Autodesk Inventor part; units mm, degrees
ref_plane "YZ Plane" through (0, 0, 0) normal (1, 0, 0) x (0, 1, 0)
ref_plane "XZ Plane" through (0, 0, 0) normal (0, 1, 0) x (-1, 0, 0)
ref_plane "XY Plane" through (0, 0, 0) normal (0, 0, 1) x (1, 0, 0)
sketch "BaseBottom" plane through (0, 0, 0) normal (0, 1, 0) x (-1, 0, 0)
  line L0 (108.8151, 0.0203) -> (-41.1849, 0.0203)
  line L1 (-46.1849, -4.9797) -> (-46.1849, -74.9797)
  line L2 (-41.1849, -79.9797) -> (108.8151, -79.9797)
  line L3 (113.8151, -74.9797) -> (113.8151, -4.9797)
  arc A0 (113.8151, -4.9797) -> (108.8151, 0.0203) centre (108.8151, -4.9797) ccw
  arc A1 (108.8151, -79.9797) -> (113.8151, -74.9797) centre (108.8151, -74.9797) ccw
  arc A2 (-46.1849, -74.9797) -> (-41.1849, -79.9797) centre (-41.1849, -74.9797) ccw
  arc A3 (-41.1849, 0.0203) -> (-46.1849, -4.9797) centre (-41.1849, -4.9797) ccw
  line L4 (109.3151, -1.9797) -> (-41.6849, -1.9797)
  line L5 (-44.1849, -4.4797) -> (-44.1849, -75.4797)
  line L6 (-41.6849, -77.9797) -> (109.3151, -77.9797)
  line L7 (111.8151, -75.4797) -> (111.8151, -4.4797)
  arc A4 (-41.6849, -1.9797) -> (-44.1849, -4.4797) centre (-41.6849, -4.4797) ccw
  arc A5 (-44.1849, -75.4797) -> (-41.6849, -77.9797) centre (-41.6849, -75.4797) ccw
  arc A6 (109.3151, -77.9797) -> (111.8151, -75.4797) centre (109.3151, -75.4797) ccw
  arc A7 (111.8151, -4.4797) -> (109.3151, -1.9797) centre (109.3151, -4.4797) ccw
  line L8 (-46.1849, -29.9797) -> (-44.1849, -29.9797)
  line L9 (-44.1849, -29.9797) -> (-44.1849, -49.9797)
  line L10 (-44.1849, -49.9797) -> (-46.1849, -49.9797)
  line L11 (-46.1849, -49.9797) -> (-46.1849, -29.9797)
  point P0 (-46.1849, -79.9797)
  point P1 (-46.1849, 0.0203)
  point P2 (113.8151, -79.9797)
  point P3 (-44.1849, -77.9797)
  point P4 (-44.1849, -1.9797)
  point P5 (111.8151, -77.9797)
  point P6 (-45.1849, -49.9797)
  dimension "d2" = 160
  dimension "d3" = 80
  dimension "d4" = 5
  dimension "d6" = 156
  dimension "d7" = 76
  dimension "d8" = 2
  dimension "d9" = 2
  dimension "d10" = 2.5
  dimension "d11" = 20
  dimension "d12" = 30
extrude "BaseFloor" add sketch "BaseBottom" against normal blind 2
extrude "BaseFill" add sketch "BaseBottom" along normal blind 98
extrude "BaseHollow" cut sketch "BaseBottom" along normal blind 100 contours L5 A4 L4 A7 L7 A6 L6 A5
properties part number "Base"
Can you work these out from the model? Positions are in its coordinate system, mm. A direction names the side the tool comes from. Give positions to 0.01 mm unless a question says otherwise; leave off trailing zeros. Write each loop counter-clockwise with the first axis right and the second up, starting at its lowest first coordinate (ties: lowest second). Pieces come first, ordered by that corner, then holes. Notation, with made-up numbers: (44.5, 28.5) -> (97.5, 28.5) arc R21 ccw to (97.5, 47.5) -> close; hole circle Ø9 at (35, 14). An arc over 180 degrees is marked (long way). Answer as a JSON object with one key per item and string values. Group by question number.
Item 1: For faces 1 (the face through (-112.389, 48.7, -1.483)), 2 (the face through (44.185, 48, -39)), which set-ups out of +Z, -Z, +X, -X, +Y, -Y let a thin tool reach every point of the face, with its end or its side?
Item 2: Suppose I cut it at A-A (y = 74.5). Please give me the cut outline in (x, z), plus the area to 3 significant figures.
Item 3: Please list where these lines run through material, in increasing order: line 1 (X direction, y = 32.5, z = -53); line 2 (Z direction, x = -41.5, y = 57); line 3 (Y direction, x = -79, z = -74.5). Write a range as [from, to].
Item 4: Suppose I cut it at B-B (z = -56). Please give me the cut outline in (x, y), plus the area to 3 significant figures.
Item 5: We'd pull the mould along Z, two halves only. Please class faces 3 (the face through (-113.815, 49, -40)), 4 (the face through (-33, 48, -77.98)), 5 (the face through (-112.312, 48.7, -78.554)): +Z half, -Z half, draft (parallel to the pull), parting line (faces both ways), or undercut.
Item 6: Suppose I cut it at C-C (x = -100). Please give me the cut outline in (y, z).
Item 7: I'm going to push a flat-ended pin straight in: P1, Ø2, axis at x = -4.5, z = -13, coming from the +Y side. Where does the tip first touch, or does it pass through?
Findings:
{
 "1": {"face 1": "+Z, -X, +Y, -Y", "face 2": "+Y"},
 "2": {"outline": "(-113.82, -74.98) arc R5 ccw to (-108.82, -79.98) -> (41.18, -79.98) arc R5 ccw to (46.18, -74.98) -> (46.18, -4.98) arc R5 ccw to (41.18, 0.02) -> (-108.82, 0.02) arc R5 ccw to (-113.82, -4.98) -> close; hole (-111.82, -75.48) arc R2.5 ccw to (-109.32, -77.98) -> (41.68, -77.98) arc R2.5 ccw to (44.18, -75.48) -> (44.18, -4.48) arc R2.5 ccw to (41.68, -1.98) -> (-109.32, -1.98) arc R2.5 ccw to (-111.82, -4.48) -> close", "area": "928 mm²"},
 "3": {"line 1": "x = [-113.82, -111.82], [44.18, 46.18]", "line 2": "z = [-79.98, -77.98], [-1.98, 0.02]", "line 3": "y = [-2, 0]"},
 "4": {"outline": "(-113.82, -2) -> (46.18, -2) -> (46.18, 98) -> (44.18, 98) -> (44.18, 0) -> (-111.82, 0) -> (-111.82, 98) -> (-113.82, 98) -> close", "area": "712 mm²"},
 "5": {"face 3": "draft", "face 4": "undercut", "face 5": "-Z half"},
 "6": {"outline": "(-2, -79.98) -> (98, -79.98) -> (98, -77.98) -> (0, -77.98) -> (0, -1.98) -> (98, -1.98) -> (98, 0.02) -> (-2, 0.02) -> close"},
 "7": {"P1": "stops at y = 0"}
}
